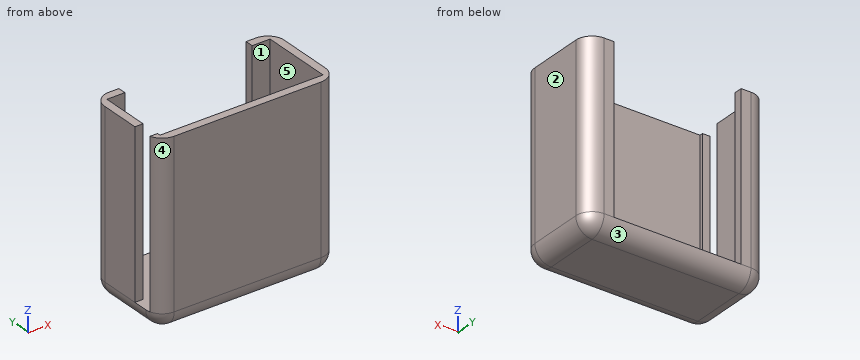
```python
from build123d import *

# Parameters (mm, degrees)
F0_W     = 39
F0_H     = 7.6218599584
F0_H_2   = 2.5
F0_W_2   = 6.4553316683
F0_H_3   = 6
F0_W_3   = 2.5
F1_DEPTH = 5
F2_DEPTH = 55
F3_R     = 4.99999


# Not quite as in the source:
# - a fillet or chamfer is up to 0.001 mm smaller than in the source, because OpenCascade refuses the exact size


with BuildPart() as f1:
    # F0 (on Top) → F1 (new body)
    with BuildSketch(Plane.XY):
        Polygon((27.5, 13.5), (19.5, 13.5), (19.5, 11), (25, 11), (25, -11), (-25, -11), (-25, -10), (-27.5, -10), (-27.5, -13.5), (27.5, -13.5), align=None)
        Polygon((-19.5, 13.5), (-27.5, 13.5), (-27.5, -4), (-25, -4), (-25, 11), (-19.5, 11), align=None)
        Polygon((-19.5, 3.3781400416), (-19.5, 11), (-25, 11), (-25, -4), (-18.5446683317, -4), (-18.5446683317, -10), (-25, -10), (-25, -11), (25, -11), (25, 11), (19.5, 11), (19.5, 3.3781400416), align=None)
        with Locations((0, 7.1890700208)):
            Rectangle(F0_W, F0_H)
        with Locations((0, 12.25)):
            Rectangle(F0_W, F0_H_2)
        with Locations((-21.7723341659, -7)):
            Rectangle(F0_W_2, F0_H_3)
        with Locations((-26.25, -7)):
            Rectangle(F0_W_3, F0_H_3)
    extrude(amount=F1_DEPTH)

    # F0 (on Top) → F2 (join)
    with BuildSketch(Plane.XY):
        Polygon((27.5, 13.5), (19.5, 13.5), (19.5, 11), (25, 11), (25, -11), (-25, -11), (-25, -10), (-27.5, -10), (-27.5, -13.5), (27.5, -13.5), align=None)
        Polygon((-19.5, 13.5), (-27.5, 13.5), (-27.5, -4), (-25, -4), (-25, 11), (-19.5, 11), align=None)
    extrude(amount=F2_DEPTH)

    # F3 (radius 5 in the source; OpenCascade refuses exactly that, so slightly less here)
    f3_edges = [f1.edges().sort_by_distance(p)[0] for p in [
        (27.5, 13.5, 27.5),
        (-27.5, 13.5, 27.5),
        (-27.5, -13.5, 27.5),
        (27.5, -13.5, 27.5),
        (-27.5, 0, 0),
        (0, 13.5, 0),
        (27.5, 0, 0),
        (0, -13.5, 0),
    ]]
    fillet(f3_edges, radius=F3_R)


solid = f1.part
```
Check sheet for the modelled part. Datum: model origin and axes. Units: mm. Face numbers are marked on the shaded views. A direction names the side the tool comes from. Give positions to 0.01 mm unless a question says otherwise; leave off trailing zeros. Write each loop counter-clockwise with the first axis right and the second up, starting at its lowest first coordinate (ties: lowest second). Pieces come first, ordered by that corner, then holes.
Item 1: Draft check along Y on the marked faces 1, 2 and 3. Enter one of: released by +Y, released by -Y, zero draft, split by the parting line, or undercut.
Item 2: Access from +Z, -Z, +X, -X, +Y, -Y to the whole of each face (thin tool, end or side, straight path). Record for the marked faces 4 and 5.
Item 3: Scan lines: L1, parallel to Y at x = 20.5, z = 42; L2, parallel to X at y = 3.75, z = 40.5; L3, parallel to X at y = -8, z = 23. Record each from-to range of solid material in increasing order.
Item 4: Cross-section at B-B (z = 49). Enter the section's corners in (x, y).
Item 5: Cross-section at D-D (y = 0.75). Enter the section's corners in (x, z).
Item 6: Gauge pin test, flat ends, axial feed: pin 1 (0.8 mm diameter, centred on y = -10.5, z = 24, fed in from +X); pin 2 (12 mm diameter, centred on x = -3.5, y = 6.5, fed in from +Z); pin 3 (1.6 mm diameter, centred on x = -23.5, z = 23.5, fed in from -Y). Record the tip position at first contact, or that the pin passes through.
Report:
1. face 1: undercut
1. face 2: zero draft
1. face 3: released by +Y
2. face 4: +Z, -Z, -X, -Y
2. face 5: +Z
3. L1: y = -13.5 to -11, 11 to 13.5
3. L2: x = -27.5 to -25, 25 to 27.5
3. L3: x = 25 to 27.5
4. outline: (-27.5, -4) - (-25, -4) - (-25, 11) - (-19.5, 11) - (-19.5, 13.5) - (-22.5, 13.5) arc R5 ccw to (-27.5, 8.5) - close; (-27.27, -10) arc R5 ccw to (-22.5, -13.5) - (22.5, -13.5) arc R5 ccw to (27.5, -8.5) - (27.5, 8.5) arc R5 ccw to (22.5, 13.5) - (19.5, 13.5) - (19.5, 11) - (25, 11) - (25, -11) - (-25, -11) - (-25, -10) - close
5. outline: (-27.5, 5) arc R5 ccw to (-22.5, 0) - (22.5, 0) arc R5 ccw to (27.5, 5) - (27.5, 55) - (25, 55) - (25, 5) - (-25, 5) - (-25, 55) - (-27.5, 55) - close
6. pin 1: stops at x = 27.24
6. pin 2: stops at z = 5
6. pin 3: stops at y = -13.5
